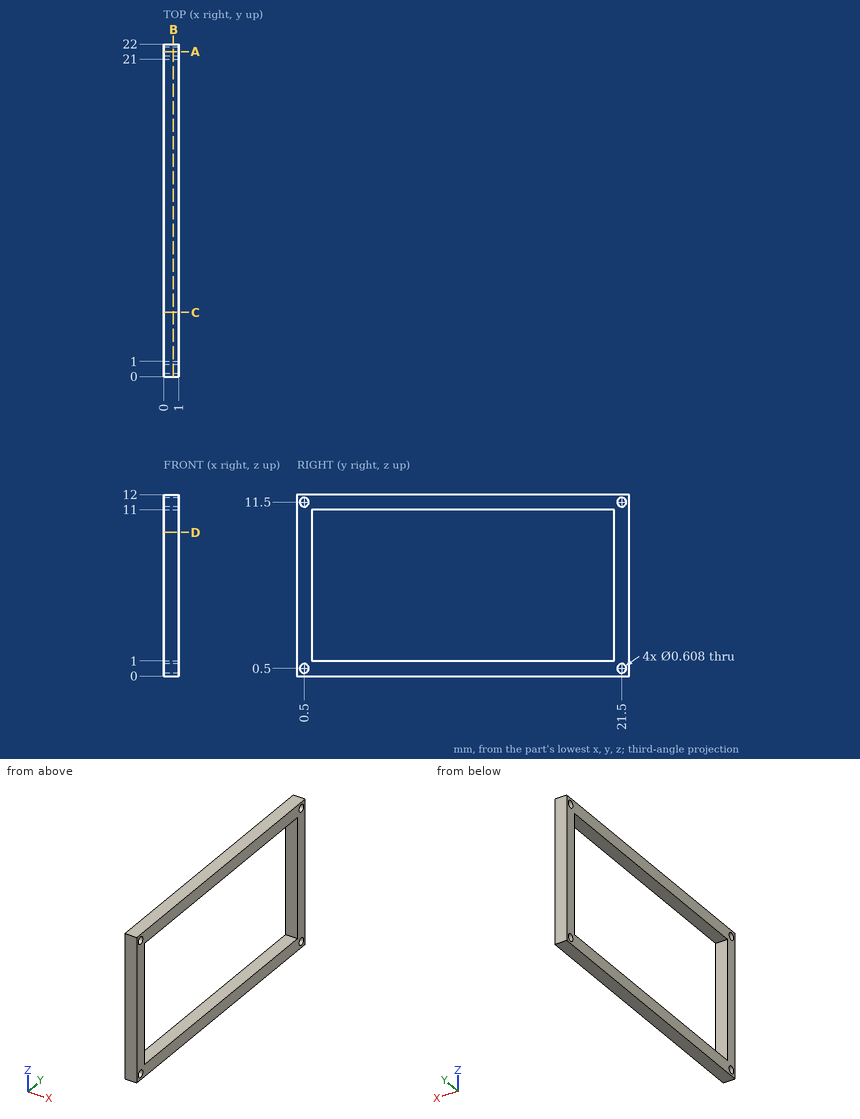
Source: three-view drawing plus pictorial views. Frame: mm from the lowest corner of the part. Coordinates: 2 decimals unless noted, no trailing zeros. Order: outer loops, then holes, each group sorted by start corner. A loop starts at its lowest first (then second) coordinate and runs counter-clockwise, first axis right, second up. Notation, with made-up numbers: M 72.5,14 L 84.5,14 A8 ccw 84.5,28 Z; hole C 19.25,60.5 d5. An arc over 180 degrees is marked long. One line per question, with ' | ' between items.
Item 1: Section C-C (y = 4.25). Output: boundary loops of the cut face in (x, z).
Geometry results:
outline: M 0,0 L 1,0 L 1,1 L 0,1 Z; M 0,11 L 1,11 L 1,12 L 0,12 Z
Item 2: Ray query, line 1 along Z through (x, y) = (0.5, 0.5) (1 decimal); line 2 along Z through (x, y) = (0.2, 5.5); line 3 along Y through (x, z) = (0.2, 1.5). Return the intervals inside material, ascending.
Geometry results:
line 1: z = 0 to 0.2, 0.8 to 11.2, 11.8 to 12 | line 2: z = 0 to 1, 11 to 12 | line 3: y = 0 to 1, 21 to 22
Item 3: Section D-D (z = 9.5). Output: boundary loops of the cut face in (x, y).
Geometry results:
outline: M 0,0 L 1,0 L 1,1 L 0,1 Z; M 0,21 L 1,21 L 1,22 L 0,22 Z
Item 4: Section A-A (y = 21.5). Give the number of separate pieces and of enclosed holes in the cut face, then the cut area to 3 significant figures.
Geometry results:
separate pieces: 3 | enclosed holes: 0 | area: 10.8 mm^2
Item 5: Section B-B (x = 0.65). Output: boundary loops of the cut face in (y, z) (1 decimal).
Geometry results:
outline: M 0,0 L 22,0 L 22,12 L 0,12 Z; hole C 0.5,0.5 d0.6; hole C 0.5,11.5 d0.6; hole M 1,1 L 21,1 L 21,11 L 1,11 Z; hole C 21.5,0.5 d0.6; hole C 21.5,11.5 d0.6
